Source: CAD feature listing. Evaluate the final solid. Frame: model axes, mm. Face numbers are marked on the shaded views. A direction names the side the tool comes from. Coordinates: 2 decimals unless noted, no trailing zeros. Write each loop counter-clockwise with the first axis right and the second up, starting at its lowest first coordinate (ties: lowest second). Pieces come first, ordered by that corner, then holes. Notation, with made-up numbers: (12.5, 60.25) - (66.5, 60.25) arc R10 ccw to (66.5, 73.25) - close; hole circle Ø1 at (87.25, 42.5). An arc over 180 degrees is marked (long way). One line per question, with ' | ' between items. Start each with the question number.
Q1. Contact query for flat-ended pins moving along their axis: P1, Ø8, axis at x = 0, y = -14.29, coming from the -Z side; P2, Ø6, axis at y = -6, z = 17, coming from the +X side; P3, Ø5, axis at y = -6, z = 12.5, coming from the -X side; P4, Ø4, axis at x = -12.37, y = 7.14, coming from the -Z side. Output: stop coordinate, or through.
Q2. Cut plane A-A, the plane x = 0. Return loops of the section in (y, z) (3 decimals).
Q3. Cut plane D-D, the plane x = 7.5. Return loops of the section in (y, z).
Q4. Draft query along X for the marked faces 1, 2, 3 and 4. Return one class per face: +X half, -X half, draft (parallel to the pull), parting line (faces both ways), or undercut.
Q5. Access query for the marked faces 5 and 6. Directions: +Z, -Z, +X, -X, +Y, -Y. A direction counts if a zero-diameter tool reaches every point of the face in a straight line with its end or side. Return the directions, or none.
Q6. Line query: line 1 (Y direction, x = 0, z = 36.3); line 2 (Z direction, x = 9, y = -7.5); line 3 (X direction, y = 4, z = 14.5). Output: solid intervals per line, ascending.
Q7. Cut plane B-B, the plane y = 0. Return loops of the section in (x, z) (3 decimals), plus the area to 3 significant figures.
Q8. Cut plane C-C, the plane y = 8. Return loops of the section in (x, z), plus the area to 3 significant figures.
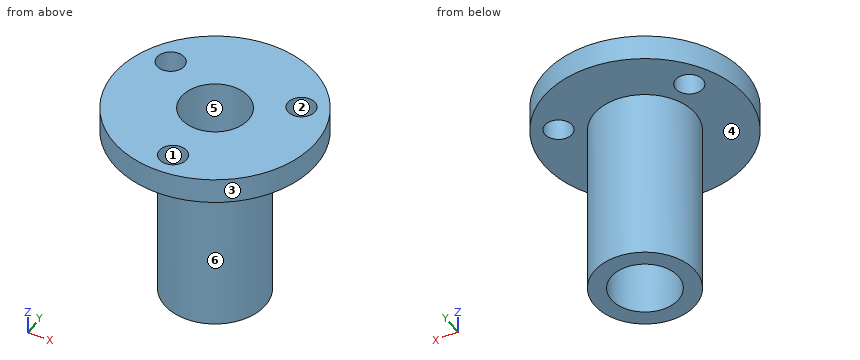
```python
from build123d import *

# Parameters (mm, degrees)
CYLINDER_R        = 9.525
CYLINDER_DEPTH    = 33.3248
SKETCH001_R       = 6.35
POCKET001_DEPTH   = 33.3258
CYLINDER001_R     = 19.05
CYLINDER001_DEPTH = 4.7752
SKETCH_R          = 2.5781
SKETCH_R_2        = 6.35
POCKET_DEPTH      = 4.7762


with BuildPart() as pocket001:
    # Cylinder → Cylinder (new body)
    with BuildSketch(Plane.XY):
        Circle(CYLINDER_R)
    extrude(amount=CYLINDER_DEPTH)

    # Sketch001 → Pocket001 (cut, through all)
    with BuildSketch(Plane(origin=(0, 0, 0), x_dir=(1, 0, 0), z_dir=(0, 0, -1))):
        Circle(SKETCH001_R)
    extrude(amount=-POCKET001_DEPTH, mode=Mode.SUBTRACT)


with BuildPart() as part:
    # Cylinder001 → Cylinder001 (new body)
    with BuildSketch(Plane.XY.offset(33.3248)):
        Circle(CYLINDER001_R)
    extrude(amount=CYLINDER001_DEPTH)

    # Sketch → Pocket (cut, through all)
    with BuildSketch(Plane.XY.offset(38.1)):
        with Locations((-12.373014, 7.144311)):
            Circle(SKETCH_R)
        with Locations((0, -14.2875)):
            Circle(SKETCH_R)
        with Locations((12.373014, 7.144311)):
            Circle(SKETCH_R)
        Circle(SKETCH_R_2)
    extrude(amount=-POCKET_DEPTH, mode=Mode.SUBTRACT)

    # Fusion: union Pocket001
    add(pocket001.part)


solid = part.part
```
Reply:
1) P1: stops at z = 33.32 | P2: stops at x = 9.04 | P3: stops at x = -8.86 | P4: passes through
2) outline: (-19.05, 33.325) - (-16.866, 33.325) - (-16.866, 38.1) - (-19.05, 38.1) - close; (-11.709, 33.325) - (-9.525, 33.325) - (-9.525, 0) - (-6.35, 0) - (-6.35, 38.1) - (-11.709, 38.1) - close; (6.35, 0) - (9.525, 0) - (9.525, 33.325) - (19.05, 33.325) - (19.05, 38.1) - (6.35, 38.1) - close
3) outline: (-17.51, 33.32) - (-5.87, 33.32) - (-5.87, 0) - (5.87, 0) - (5.87, 33.32) - (17.51, 33.32) - (17.51, 38.1) - (-17.51, 38.1) - close
4) face 1: undercut | face 2: undercut | face 3: parting line | face 4: draft
5) face 5: +Z, -Z | face 6: -Z
6) line 1: y = -19.05 to -16.87, -11.71 to -6.35, 6.35 to 19.05 | line 2: z = 33.32 to 38.1 | line 3: x = -8.64 to -4.93, 4.93 to 8.64
7) outline: (-19.05, 33.325) - (-9.525, 33.325) - (-9.525, 0) - (-6.35, 0) - (-6.35, 38.1) - (-19.05, 38.1) - close; (6.35, 0) - (9.525, 0) - (9.525, 33.325) - (19.05, 33.325) - (19.05, 38.1) - (6.35, 38.1) - close | area: 333 mm^2
8) outline: (-17.29, 33.32) - (-14.8, 33.32) - (-14.8, 38.1) - (-17.29, 38.1) - close; (-9.94, 33.32) - (-5.17, 33.32) - (-5.17, 0) - (5.17, 0) - (5.17, 33.32) - (9.94, 33.32) - (9.94, 38.1) - (-9.94, 38.1) - close; (14.8, 33.32) - (17.29, 33.32) - (17.29, 38.1) - (14.8, 38.1) - close | area: 463 mm^2
